Could you check a few things on this model? Use its own coordinates, in mm. A direction names the side the tool comes from. Coordinates: 2 decimals unless noted, no trailing zeros. Write each loop counter-clockwise with the first axis right and the second up, starting at its lowest first coordinate (ties: lowest second). Pieces come first, ordered by that corner, then holes.
```python
from build123d import *

# Parameters (mm, degrees)
F2_DEPTH = 1
F3_DEPTH = 50.5
F4_SIZE  = 1.2
F5_SIZE  = 0.9
F7_DEPTH = 1


with BuildPart() as f2:
    # F1 (on Top) → F2 (new body)
    with BuildSketch(Plane.XY):
        with BuildLine():
            Line((0, 0), (-4, 0))
            Line((-4, 0), (-4, -13.8431457505))
            Line((-4, -13.8431457505), (-28.25, -38.0931457505))
            Line((-28.25, -38.0931457505), (-28.25, -40.75))
            ThreePointArc((-28.25, -40.75), (-27.3713203436, -42.8713203436), (-25.25, -43.75))
            Line((-25.25, -43.75), (-22.5931457505, -43.75))
            Line((-22.5931457505, -43.75), (0, -21.1568542495))
            Line((0, -21.1568542495), (0, 0))
        make_face()
        with BuildLine():
            Line((-28.25, -40.75), (-28.25, -38.0931457505))
            Line((-28.25, -38.0931457505), (-29.45, -39.2931457505))
            Line((-29.45, -39.2931457505), (-29.45, -40.75))
            ThreePointArc((-29.45, -40.75), (-28.219848481, -43.719848481), (-25.25, -44.95))
            Line((-25.25, -44.95), (-23.7931457505, -44.95))
            Line((-23.7931457505, -44.95), (-22.5931457505, -43.75))
            Line((-22.5931457505, -43.75), (-25.25, -43.75))
            ThreePointArc((-25.25, -43.75), (-27.3713203436, -42.8713203436), (-28.25, -40.75))
        make_face()
    extrude(amount=-F2_DEPTH)

    # F1 (on Top) → F3 (join)
    with BuildSketch(Plane.XY):
        with BuildLine():
            Line((-28.25, -40.75), (-28.25, -38.0931457505))
            Line((-28.25, -38.0931457505), (-29.45, -39.2931457505))
            Line((-29.45, -39.2931457505), (-29.45, -40.75))
            ThreePointArc((-29.45, -40.75), (-28.219848481, -43.719848481), (-25.25, -44.95))
            Line((-25.25, -44.95), (-23.7931457505, -44.95))
            Line((-23.7931457505, -44.95), (-22.5931457505, -43.75))
            Line((-22.5931457505, -43.75), (-25.25, -43.75))
            ThreePointArc((-25.25, -43.75), (-27.3713203436, -42.8713203436), (-28.25, -40.75))
        make_face()
    extrude(amount=F3_DEPTH)

    # F4
    f4_edges = [f2.edges().sort_by_distance(p)[0] for p in [
        (-28.25, -38.093146, 25.25),
        (-22.593146, -43.75, 25.25),
    ]]
    chamfer(f4_edges, length=F4_SIZE)

    # F5
    f5_edges = [f2.edges().sort_by_distance(p)[0] for p in [
        (-23.61741, -44.174264, 0),
        (-28.674264, -39.11741, 0),
    ]]
    chamfer(f5_edges, length=F5_SIZE)

    # F6 (on face) → F7 (join)
    with BuildSketch(Plane.XY.offset(50.5)):
        with BuildLine():
            Line((-25.25, -43.75), (-23.7931457505, -43.75))
            Line((-23.7931457505, -43.75), (-28.25, -39.2931457505))
            Line((-28.25, -39.2931457505), (-28.25, -40.75))
            ThreePointArc((-28.25, -40.75), (-27.3713203436, -42.8713203436), (-25.25, -43.75))
        make_face()
        with BuildLine():
            Line((-23.4416738879, -44.5985281374), (-23.7931457505, -43.75))
            Line((-23.7931457505, -43.75), (-25.25, -43.75))
            ThreePointArc((-25.25, -43.75), (-27.3713203436, -42.8713203436), (-28.25, -40.75))
            Line((-28.25, -40.75), (-28.25, -39.2931457505))
            Line((-28.25, -39.2931457505), (-29.0985281374, -38.9416738879))
            Line((-29.0985281374, -38.9416738879), (-29.45, -39.2931457505))
            Line((-29.45, -39.2931457505), (-29.45, -40.75))
            ThreePointArc((-29.45, -40.75), (-28.219848481, -43.719848481), (-25.25, -44.95))
            Line((-25.25, -44.95), (-23.7931457505, -44.95))
            Line((-23.7931457505, -44.95), (-23.4416738879, -44.5985281374))
        make_face()
    extrude(amount=F7_DEPTH)

    # F8: F2 across face


with BuildPart() as f2_1:
    add(f2.part)
    add(f2.part.mirror(Plane(origin=(0, -10.5784271247, -0.5), x_dir=(0, 1, 0), z_dir=(1, 0, 0))))

    # F9: F2 across face


with BuildPart() as f2_2:
    add(f2_1.part)
    add(f2_1.part.mirror(Plane(origin=(0, 0, -0.5), x_dir=(-1, 0, 0), z_dir=(0, 1, 0))))


solid = f2_2.part
```
Item 1: Will these pins go through, and if not, where does the flat tip stop? pin 1 Ø1.5 at (x, y) = (2.5, -10.5) entering from +Z; pin 2 Ø10 at (x, z) = (15.5, 28.5) entering from -Y; pin 3 Ø0.5 at (y, z) = (3.5, -0.5) entering from -X.
Item 2: I want a section at A-A, the plane y = -23. List the corners of the cut face in (x, z) for me, then the cut area to 3 significant figures.
Item 3: Which directions (+Z, -Z, +X, -X, +Y, -Y) give clear straight access to the entire face, cutting with the end or side of a thin tool? Please do faces 1 (the flat face through (-16.666, -26.509, -0.15)), 2 (the flat face through (11.952, 33.109, -0.15)), 3 (the cylindrical face through (-27.35, 42.89, 24.9)).
Item 4: If we mould it in two halves opening along Z, with no side actions, what happens to faces 4 (the flat face through (-27, 43, 51.5)), 5 (the flat face through (-11.952, -33.109, -0.15)), 6 (the flat face through (-25, -43.75, 25)), 7 (the flat face through (-27, 42, 50.5))? For each: released by +Z, released by -Z, zero draft, split by the parting line, or undercut.
Item 5: I want a section at C-C, the plane x = 12. List the corners of the cut face in (y, z) for me.
Item 6: If I drill on line 1 along X through (y, z) = (40, 39); line 2 along Y through (x, z) = (-27, 20); line 3 along Z through (x, y) = (-22, 37), over which ranges is the centre line in solid material (lowest first)?
Item 7: I want a section at B-B, the plane z = 24. Count the separate pieces of the cut face and the enclosed holes in it, then the cut area to 3 significant figures.
Item 8: I want a section at D-D, the plane x = 1. List the corners of the cut face in (y, z) for me, then the cut area to 3 significant figures.
Taken from the geometry:
1. pin 1: stops at z = 0
1. pin 2: passes through
1. pin 3: stops at x = -4
2. outline: (-13.16, -1) - (-1.84, -1) - (-1.84, 0) - (-13.16, 0) - close; (1.84, -1) - (13.16, -1) - (13.16, 0) - (1.84, 0) - close
2. area: 22.6 mm2
3. face 1: +Z, -Z, -X
3. face 2: +Z, -Z, +Y
3. face 3: none
4. face 4: released by +Z
4. face 5: zero draft
4. face 6: undercut
4. face 7: undercut
5. outline: (-33.16, -1) - (-21.84, -1) - (-21.84, 0) - (-33.16, 0) - close; (21.84, -1) - (33.16, -1) - (33.16, 0) - (21.84, 0) - close
6. line 1: x = -29.45 to -28.25, 28.25 to 29.45
6. line 2: y = -44.57 to -43.19, 43.19 to 44.57
6. line 3: z = -1 to 0
7. separate pieces: 4
7. enclosed holes: 0
7. area: 42.8 mm2
8. outline: (-22.16, -1) - (22.16, -1) - (22.16, 0) - (-22.16, 0) - close
8. area: 44.3 mm2
